Could you check a few things on this model? Use its own coordinates, in mm. Coordinates: 2 decimals unless noted, no trailing zeros. Loops run counter-clockwise (first coordinate to the right, second up) from the corner with the lowest first, then second, coordinate; pieces in that order, holes last.
Autodesk Inventor part; units mm, degrees
ref_plane "YZ Plane" through (0, 0, 0) normal (1, 0, 0) x (0, 1, 0)
ref_plane "XZ Plane" through (0, 0, 0) normal (0, 1, 0) x (-1, 0, 0)
ref_plane "XY Plane" through (0, 0, 0) normal (0, 0, 1) x (1, 0, 0)
sketch "Sketch1" plane through (0, 0, 0) normal (0, 1, 0) x (-1, 0, 0)
  circle A0 centre (0, 0) radius 6.15
  line L0 (0, -9.2376) -> (-8, -4.6188)
  line L1 (-8, -4.6188) -> (-8, 4.6188)
  line L2 (-8, 4.6188) -> (0, 9.2376)
  line L3 (0, 9.2376) -> (8, 4.6188)
  line L4 (8, 4.6188) -> (8, -4.6188)
  line L5 (8, -4.6188) -> (0, -9.2376)
  dimension "d0" = 12.3
  dimension "d1" = 16
extrude "Extrusion1" add sketch "Sketch1" along normal blind 2
thread "Thread1"
properties part number "Switch Nut"
1) Imagine slicing it at C-C on x = -2.5. List the corners of the cut face in (y, z) for me, plus the area to 3 significant figures.
2) Imagine slicing it at B-B on z = 0. List the corners of the cut face in (x, y) for me.
3) Imagine slicing it at D-D on z = -6.5. List the corners of the cut face in (x, y) for me, plus the area to 3 significant figures.
4) Will this pin go through, and if not, where does the flat tip stop? pin 1 (5 mm diameter, centred on x = 1, z = -2.5, fed in from -Y).
5) We'd pull the mould along Z, two halves only. Please class faces 1 (the flat face through (3.944, 0.986, -6.961)), 2 (the flat face through (-8, 1, 0)), 3 (the cylindrical face through (1.333, 0.986, 6.004)): released by +Z, released by -Z, zero draft, split by the parting line, or undercut.
6) Imagine slicing it at A-A on y = 1.6. List the corners of the cut face in (x, z) for me, plus the area to 3 significant figures.
7) If I drill on L1, parallel to X at y = 0.5, z = 3.75; L2, parallel to Z at x = 5, y = 1.95; L3, parallel to X at y = 1.9, z = 3, over which ranges is the centre line in solid material (lowest first)?
Solved:
1. outline: (0, -7.79) - (2, -7.79) - (2, -5.62) - (0, -5.62) - close; (0, 5.62) - (2, 5.62) - (2, 7.79) - (0, 7.79) - close
1. area: 8.70 mm2
2. outline: (-8, 0) - (-6.15, 0) - (-6.15, 2) - (-8, 2) - close; (6.15, 0) - (8, 0) - (8, 2) - (6.15, 2) - close
3. outline: (-4.74, 0) - (4.74, 0) - (4.74, 2) - (-4.74, 2) - close
3. area: 19.0 mm2
4. pin 1: passes through
5. face 1: released by -Z
5. face 2: zero draft
5. face 3: undercut
6. outline: (-8, -4.62) - (0, -9.24) - (8, -4.62) - (8, 4.62) - (0, 9.24) - (-8, 4.62) - close; hole circle Ø12.3 at (0, 0)
6. area: 103 mm2
7. L1: x = -8 to -4.87, 4.87 to 8
7. L2: z = -6.35 to -3.58, 3.58 to 6.35
7. L3: x = -8 to -5.37, 5.37 to 8
